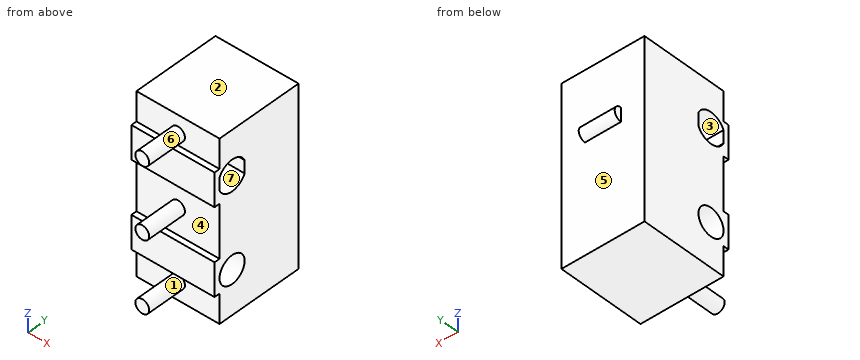
from build123d import *

# Parameters (mm, degrees)
SKETCH090_R             = 1
PAD055_DEPTH            = 6
CYLINDER080_R           = 0.5
CYLINDER080_DEPTH       = 3
LINEARPATTERN001_COUNT  = 3
LINEARPATTERN001_PITCH  = 5.1
CYLINDER081_R           = 0.5
CYLINDER081_DEPTH       = 2.6
BODY073_PITCH_ANGLE     = 88.936822
BODY073_PLACEMENT_ANGLE = -90
BODY074_ROLL_ANGLE      = 1.063178
BODY074_PLACEMENT_ANGLE = -90
BODY075_PLACEMENT_ANGLE = 90
BODY076_PLACEMENT_ANGLE = 90


with BuildPart() as part:
    # Sketch090 → Pad055 (new body)
    with BuildSketch(Plane.XY):
        Polygon((6.4, 3.15), (6.4, -3.15), (4.3, -3.15), (4.3, -3.55), (1.9, -3.55), (1.9, -3.15), (-1.9, -3.15), (-1.9, -3.55), (-4.3, -3.55), (-4.3, -3.15), (-6.4, -3.15), (-6.4, 3.15), (-3.4, 3.15), align=None)
        with Locations((3.25, -2.15)):
            Circle(SKETCH090_R, mode=Mode.SUBTRACT)
        with BuildLine():
            ThreePointArc((-3.708258, -1.15), (-4.35, -2.15), (-3.708258, -3.15))
            Line((-2.791742, -3.15), (-3.708258, -3.15))
            ThreePointArc((-2.791742, -3.15), (-2.15, -2.15), (-2.791742, -1.15))
            Line((-3.708258, -1.15), (-2.791742, -1.15))
        make_face(mode=Mode.SUBTRACT)
    extrude(amount=PAD055_DEPTH)

    # Cylinder080 → Cylinder080 (join)
    with BuildSketch(Plane(origin=(-5.1, -3, 3), x_dir=(1, 0, 0), z_dir=(0, -1, 0))):
        Circle(CYLINDER080_R)
    cylinder080 = extrude(amount=CYLINDER080_DEPTH)

    # LinearPattern001: Cylinder080 ×3
    with Locations(*[(i * LINEARPATTERN001_PITCH, 0, 0) for i in range(1, LINEARPATTERN001_COUNT)]):
        add(cylinder080)

    # Cylinder081 → Cylinder081 (join)
    with BuildSketch(Plane(origin=(-1.9, 3.15, 1.7), x_dir=(1, 0, 0), z_dir=(0, 0, 1))):
        Circle(CYLINDER081_R)
    extrude(amount=CYLINDER081_DEPTH)


with BuildPart() as part_1:
    # Body073 pitch: moved
    add(part.part.rotate(Axis((0, 0, 0), (0, 1, 0)), BODY073_PITCH_ANGLE))


with BuildPart() as part_2:
    # Body073 placement: moved
    add(part_1.part.moved(Location((-7.15, 2.882282, 8.601102))).rotate(Axis((-7.15, 2.882282, 8.601102), (0, 0, 1)), BODY073_PLACEMENT_ANGLE))


with BuildPart() as part_3:
    # Body074 roll: moved
    add(part_2.part.rotate(Axis((0, 0, 0), (1, 0, 0)), BODY074_ROLL_ANGLE))


with BuildPart() as part_4:
    # Body074 placement: moved
    add(part_3.part.moved(Location((0.277807, 0, -0.053101))).rotate(Axis((0.277807, 0, -0.053101), (0, 0, 1)), BODY074_PLACEMENT_ANGLE))


with BuildPart() as part_5:
    # Body075 placement: moved
    add(part_4.part.moved(Location((0, 0.105928, 0))).rotate(Axis((0, 0.105928, 0), (0, 0, -1)), BODY075_PLACEMENT_ANGLE))


with BuildPart() as part_6:
    # Body076 placement: moved
    add(part_5.part.moved(Location((-0.105928, 0, 0))).rotate(Axis((-0.105928, 0, 0), (0, 0, -1)), BODY076_PLACEMENT_ANGLE))


solid = part_6.part
Can you work these out from the model? Positions are in its coordinate system, mm. Face numbers are marked on the shaded views. A direction names the side the tool comes from. Give positions to 0.01 mm unless a question says otherwise; leave off trailing zeros. Loops run counter-clockwise (first coordinate to the right, second up) from the corner with the lowest first, then second, coordinate; pieces in that order, holes last. Notation, with made-up numbers: M -35,-6 L 11,-6 A31 cw 11,29 Z; hole C 4.25,50.5 d5. An arc over 180 degrees is marked long. One line per item, written item: value. Start each with the question number.
1) I'm going to push flat-ended pins straight in: pin 1 (1 mm diameter, centred on x = -2, z = 7.5, fed in from +Y); pin 2 (1.2 mm diameter, centred on x = -1, z = 6, fed in from -Y). Where does each tip first touch, or does it pass through?
2) Thinking about a two-plate mould opening in Y: for the marked faces 4, 5, 6 and 7, which applies, +Y half, -Y half, draft (parallel to the pull), parting line (faces both ways), or undercut?
3) If I drill on line 1 (Z direction, x = 0, y = -11.5); line 2 (Y direction, x = -0.55, z = 5.35); line 3 (X direction, y = -11.5, z = 13.75), over which ranges is the centre line in solid material (lowest first)? Write a range as [from, to].
4) On a 3-axis mill with a long thin cutter (end or side, diameter ignored), from which of +Z, -Z, +X, -X, +Y, -Y can I reach the whole of each face in a straight line? I mean the marked faces 1, 2 and 3. Say none if no direction works.
5) If we section it at B-B, the plane y = -9.3: Write out the boundary of the cut face in (x, z), and give its area (3 significant figures).
6) If we section it at D-D, the plane z = 3.5: Write out the boundary of the cut face in (x, y).
7) If we section it at C-C, the plane x = -0.75: Write out the boundary of the cut face in (y, z).
8) If we section it at A-A, the plane z = 5.35: Write out the boundary of the cut face in (x, y), and give its area (3 significant figures).
Completed:
1. pin 1: stops at y = -4
1. pin 2: stops at y = -10.7
2. face 4: -Y half
2. face 5: +Y half
2. face 6: draft
2. face 7: undercut
3. line 1: z = [3, 4], [8.1, 9.1], [13.2, 14.2]
3. line 2: y = [-10.7, -10.3], [-8.3, -4]
3. line 3: x = [-0.5, 0.5]
4. face 1: -Y
4. face 2: +Z, +X, -X, +Y, -Y
4. face 3: +X, -X
5. outline: M -3,2.2 L 3,2.2 L 3,4.35 L -3,4.35 Z; M -3,6.35 L 3,6.35 L 3,10.75 L -3,10.75 Z; M -3,12.95 L 3,12.95 L 3,15 L -3,15 Z
5. area: 51.6 mm^2
6. outline: M -3,-10.3 L -0.5,-10.3 L -0.5,-13.15 L 0.5,-13.15 L 0.5,-10.3 L 3,-10.3 L 3,-4 L -3,-4 Z
7. outline: M -10.7,4.3 L -10.3,4.3 L -10.3,2.2 L -4,2.2 L -4,10 A0.5 ccw -4,11 L -4,15 L -10.3,15 L -10.3,12.9 L -10.7,12.9 L -10.7,10.5 L -10.3,10.5 L -10.3,6.7 L -10.7,6.7 Z; hole C -9.3,5.35 d2; hole M -10.3,11.39 A1.1 ccw -8.3,11.39 L -8.3,12.31 A1.1 ccw -10.3,12.31 Z
8. outline: M -3,-10.7 L 3,-10.7 L 3,-10.3 L -3,-10.3 Z; M -3,-8.3 L 3,-8.3 L 3,-4 L -3,-4 Z
8. area: 28.2 mm^2
